Here's how the part is built. I have some questions about the finished solid (model axes, mm). A direction names the side the tool comes from. Round coordinates to 2 decimals unless told otherwise and drop trailing zeros. Loops run counter-clockwise (first coordinate to the right, second up) from the corner with the lowest first, then second, coordinate; pieces in that order, holes last. Notation, with made-up numbers: (47, 70) - (90, 70) arc R21 ccw to (90, 94) - close; hole circle Ø2 at (-13, 38.25). An arc over 180 degrees is marked (long way). Answer as a JSON object with one key per item and string values. Group by question number.
1) Which directions (+Z, -Z, +X, -X, +Y, -Y) give clear straight access to the entire face, cutting with the end or side of a thin tool? Please do faces 4 (the face through (4.5, 0.5, -2.927)), 5 (the face through (-3.872, 3, -5.2)), 6 (the face through (0.05, 0.92, -3.62)).
2) I want a section at A-A, the plane x = -4. Please give me the cut outline in (y, z), then the cut area to 3 significant figures.
3) Will these pins go through, and if not, where does the flat tip stop? P1, Ø1.5, axis at x = 1, y = 3.5, coming from the +Z side; P2, Ø0.6, axis at y = 0, z = -0.5, coming from the +X side; P3, Ø1, axis at x = 2, z = -3.5, coming from the +Y side.
4) I want a section at D-D, the plane x = -2.75. Please give me the cut outline in (y, z).
5) If I drill on line 1 along X through (y, z) = (0.25, -1); line 2 along Z through (x, y) = (3.75, 0.75); line 3 along Y through (x, z) = (-0.5, -1), over which ranges is the centre line in solid material (lowest first)? Write a range as [from, to].
6) I want a section at C-C, the plane y = 2.5. Please give me the cut outline in (x, z), then the cut area to 3 significant figures.
7) If we mould it in two halves opening along Z, with no side actions, what happens to faces 1 (the face through (3.872, 3, -5.2)), 2 (the face through (0, 0, 1.185)), 3 (the face through (0, -0.422, -1))? For each: pulls with the +Z half, pulls with the -Z half, needs draft (parallel to the pull), parting line crosses it, or undercut.
from build123d import *

# Parameters (mm, degrees)
SKETCH51_W           = 6.2865
SKETCH51_H           = 2.794
BOSS_EXTRUDE23_DEPTH = 7.8
SKETCH49_W           = 1.143
SKETCH49_H           = 1.143
CUT_EXTRUDE22_DEPTH  = 9.861515478
BOSS_EXTRUDE24_DEPTH = 5.92
SKETCH52_W           = 0.635
SKETCH52_H           = 0.889
SKETCH52_W_2         = 1.4224
BOSS_EXTRUDE25_DEPTH = 0.508
SCALE1_SCALE         = 0.654


with BuildPart() as part:
    # Sketch51 → Boss-Extrude23 (new, symmetric)
    with BuildSketch(Plane(origin=(0, 0, 0), x_dir=(0, 0, -1), z_dir=(1, 0, 0))):
        Rectangle(SKETCH51_W, SKETCH51_H)
    extrude(amount=BOSS_EXTRUDE23_DEPTH, both=True)

    # Sketch49 → Cut-Extrude22 (cut, through all)
    with BuildSketch(Plane(origin=(0, 1.397, 0), x_dir=(1, 0, 0), z_dir=(0, 1, 0))):
        with Locations((1.9812, -0.003489448)):
            Rectangle(SKETCH49_W, SKETCH49_H)
        with Locations((5.9436, -0.003489448)):
            Rectangle(SKETCH49_W, SKETCH49_H)
        with Locations((-1.9812, -0.003489448)):
            Rectangle(SKETCH49_W, SKETCH49_H)
        with Locations((-5.9436, -0.003489448)):
            Rectangle(SKETCH49_W, SKETCH49_H)
    extrude(amount=-CUT_EXTRUDE22_DEPTH, mode=Mode.SUBTRACT)

    # Sketch50 → Boss-Extrude24 (add, symmetric)
    with BuildSketch(Plane(origin=(0, 0, 0), x_dir=(0, 0, -1), z_dir=(1, 0, 0))):
        with BuildLine():
            Line((3.14325, -1.905), (5.08635, -1.905))
            ThreePointArc((5.08635, -1.905), (6.343585857, -1.384235857), (6.86435, -0.127))
            Line((6.86435, -0.127), (6.86435, 9.4234))
            Line((6.86435, 9.4234), (6.22935, 9.4234))
            Line((6.22935, 9.4234), (4.509763171, 7.222429228))
            ThreePointArc((4.509763171, 7.222429228), (4.409745704, 7.038219969), (4.37515, 6.831484191))
            Line((4.37515, 6.831484191), (4.37515, 6.655190003))
            ThreePointArc((4.37515, 6.655190003), (4.423486497, 6.412186024), (4.561137194, 6.206177197))
            Line((4.561137194, 6.206177197), (5.857375612, 4.909938779))
            ThreePointArc((5.857375612, 4.909938779), (6.132677006, 4.497921126), (6.22935, 4.011913167))
            Line((6.22935, 4.011913167), (6.22935, 0.455913167))
            ThreePointArc((6.22935, 0.455913167), (5.887560369, -0.107338712), (5.230128963, -0.064248381))
            Line((5.230128963, -0.064248381), (3.14325, 1.397))
            Line((3.14325, 1.397), (3.14325, -1.905))
        make_face()
    extrude(amount=BOSS_EXTRUDE24_DEPTH, both=True)

    # Sketch52 → Boss-Extrude25 (add)
    with BuildSketch(Plane(origin=(0, -1.397, 0), x_dir=(1, 0, 0), z_dir=(0, 1, 0))):
        with Locations((7.5311, -2.69875)):
            Rectangle(SKETCH52_W, SKETCH52_H)
        with Locations((0, -2.69875)):
            Rectangle(SKETCH52_W_2, SKETCH52_H)
        with Locations((3.9624, -2.69875)):
            Rectangle(SKETCH52_W_2, SKETCH52_H)
        with Locations((-3.9624, -2.69875)):
            Rectangle(SKETCH52_W_2, SKETCH52_H)
        with Locations((-7.5311, -2.69875)):
            Rectangle(SKETCH52_W, SKETCH52_H)
    extrude(amount=-BOSS_EXTRUDE25_DEPTH)


with BuildPart() as part_1:
    # Scale1: scaled about (0, 1.420456249, -2.517201016)
    add(part.part.scale(SCALE1_SCALE).moved(Location((0, 0.491477862, -0.870951552))))


solid = part_1.part
Outcome:
{
 "1": {"face 4": "-Z, +X, +Y, -Y", "face 5": "-Z, -X, +Y, -Y", "face 6": "+X, -X"},
 "2": {"outline": "(-0.42, -2.93) - (1.41, -2.93) - (1.41, -1.24) - (-0.42, -1.24) - close; (-0.42, -0.49) - (1.41, -0.49) - (1.41, 1.18) - (-0.42, 1.18) - close", "area": "6.15 mm^2"},
 "3": {"P1": "z = -4.15", "P2": "x = 5.1", "P3": "y = 5.44"},
 "4": {"outline": "(-0.75, -4.2) arc R1.16 ccw to (0.41, -5.36) - (6.65, -5.36) - (6.65, -4.94) - (5.21, -3.82) arc R0.42 ccw to (4.96, -3.73) - (4.84, -3.73) arc R0.42 ccw to (4.55, -3.85) - (3.7, -4.7) arc R0.83 cw to (3.12, -4.94) - (0.79, -4.94) arc R0.42 cw to (0.45, -4.29) - (1.41, -2.93) - (1.41, 1.18) - (-0.75, 1.18) - (-0.75, 0.6) - (-0.42, 0.6) - (-0.42, -2.93) - (-0.75, -2.93) - close"},
 "5": {"line 1": "[-5.1, -4.26], [-3.51, -1.67], [-0.92, 0.92], [1.67, 3.51], [4.26, 5.1]", "line 2": "[-5.36, -4.94], [-3.86, -1.24], [-0.49, 1.18]", "line 3": "[-0.42, 1.41]"},
 "6": {"outline": "(-3.87, -5.36) - (3.87, -5.36) - (3.87, -4.94) - (-3.87, -4.94) - close", "area": "3.22 mm^2"},
 "7": {"face 1": "needs draft", "face 2": "pulls with the +Z half", "face 3": "undercut"}
}
